from build123d import *

# Parameters (mm, degrees)
F0_W     = 80
F0_H     = 40
F1_DEPTH = 5
F2_W     = 80
F2_H     = 25
F2_R     = 3
F3_DEPTH = 5
F4_R     = 4.99999
F5_R     = 3
F6_DEPTH = 3


# Not quite as in the source:
# - a fillet or chamfer is up to 0.001 mm smaller than in the source, because OpenCascade refuses the exact size


with BuildPart() as f1:
    # F0 (on Top) → F1 (new body)
    with BuildSketch(Plane.XY):
        with Locations((-1.6386443377, -15.6908366084)):
            Rectangle(F0_W, F0_H)
    extrude(amount=-F1_DEPTH)

    # F2 (on face) → F3 (join)
    with BuildSketch(Plane.XZ.offset(35.6908366084)):
        with Locations((-1.6386443377, 12.5)):
            Rectangle(F2_W, F2_H)
        with Locations((-11.1386443377, 10)):
            Circle(F2_R, mode=Mode.SUBTRACT)
        with Locations((7.8613556623, 10)):
            Circle(F2_R, mode=Mode.SUBTRACT)
    extrude(amount=-F3_DEPTH)

    # F4 (radius 5 in the source; OpenCascade refuses exactly that, so slightly less here)
    f4_edges = [f1.edges().sort_by_distance(p)[0] for p in [
        (-41.638644, -33.190837, 25),
        (38.361356, -33.190837, 25),
        (-1.638644, 4.309163, 0),
    ]]
    fillet(f4_edges, radius=F4_R)

    # F5 (on face) → F6 (cut)
    with BuildSketch(Plane(origin=(0, -30.6908366084, 0), x_dir=(-1, 0, 0), z_dir=(0, 1, 0))):
        with BuildLine():
            ThreePointArc((-7.8613556623, 1.5), (-1.8509480223, 3.9895923599), (0.6386443377, 10))
            ThreePointArc((0.6386443377, 10), (-1.8509480223, 16.0104076401), (-7.8613556623, 18.5))
            ThreePointArc((-7.8613556623, 18.5), (-16.3613556623, 10), (-7.8613556623, 1.5))
        make_face()
        with Locations((-7.8613556623, 10)):
            Circle(F5_R, mode=Mode.SUBTRACT)
        with BuildLine():
            ThreePointArc((-7.8613556623, 18.5), (-1.8509480223, 16.0104076401), (0.6386443377, 10))
            ThreePointArc((0.6386443377, 10), (-1.8509480223, 3.9895923599), (-7.8613556623, 1.5))
            Line((-7.8613556623, 1.5), (11.1386443377, 1.5))
            ThreePointArc((11.1386443377, 1.5), (2.6386443377, 10), (11.1386443377, 18.5))
            Line((11.1386443377, 18.5), (-7.8613556623, 18.5))
        make_face()
        with BuildLine():
            ThreePointArc((19.6386443377, 10), (17.1490519777, 16.0104076401), (11.1386443377, 18.5))
            ThreePointArc((11.1386443377, 18.5), (2.6386443377, 10), (11.1386443377, 1.5))
            ThreePointArc((11.1386443377, 1.5), (17.1490519777, 3.9895923599), (19.6386443377, 10))
        make_face()
        with Locations((11.1386443377, 10)):
            Circle(F5_R, mode=Mode.SUBTRACT)
        with Locations((11.1386443377, 10)):
            Circle(F5_R)
        with Locations((-7.8613556623, 10)):
            Circle(F5_R)
    extrude(amount=-F6_DEPTH, mode=Mode.SUBTRACT)


solid = f1.part
Source: CAD feature listing. Evaluate the final solid. Frame: model axes, mm. A direction names the side the tool comes from. Round coordinates to 2 decimals unless told otherwise and drop trailing zeros. Loops run counter-clockwise (first coordinate to the right, second up) from the corner with the lowest first, then second, coordinate; pieces in that order, holes last.
Q1. Section A-A, the plane y = -32. Return loops of the section in (x, z).
Q2. First-contact query: P1, Ø24, axis at x = -11, y = -16.5, coming from the +Z side; P2, Ø5, axis at x = -2, z = 7.5, coming from the +Y side; P3, Ø4, axis at x = 8, z = 17, coming from the +Y side. Flat tips, straight axial feed; report the tip coordinate or a pass-through.
Q3. Mould query, pull axis Z, two halves, no side actions, for faces 4 (the face through (-2, -32, 18.5)), 5 (the face through (-1.08, 2.81, -1.43)), 6 (the face through (-41.639, -23, -1)). Classes: pulls with the +Z half, pulls with the -Z half, needs draft (parallel to the pull), parting line crosses it, or undercut.
Q4. Access query for faces 1 (the face through (-2, -15, 0)), 2 (the face through (-40.21, -33.16, 23.5)), 3 (the face through (-1, -33.691, 10)). Directions: +Z, -Z, +X, -X, +Y, -Y. A direction counts if a zero-diameter tool reaches every point of the face in a straight line with its end or side. Return the directions, or none.
Q5. Ray query, line 1 (Y direction, x = -24, z = 6.25); line 2 (Z direction, x = 12.5, y = -27.5); line 3 (Y direction, x = 5.5, z = 15.25). Return the intervals inside material, ascending.
Q6. Section D-D, the plane z = 14. Return loops of the section in (x, y).
Q7. Section C-C, the plane z = 9. Return loops of the section in (x, y), plus the area to 3 significant figures.
Solutions:
1. outline: (-41.64, -5) - (38.36, -5) - (38.36, 20) arc R5 ccw to (33.36, 25) - (-36.64, 25) arc R5 ccw to (-41.64, 20) - close; hole (-11.14, 1.5) - (7.86, 1.5) arc R8.5 ccw to (7.86, 18.5) - (-11.14, 18.5) arc R8.5 ccw to start
2. P1: stops at z = 0
2. P2: stops at y = -33.69
2. P3: stops at y = -30.69
3. face 4: undercut
3. face 5: pulls with the +Z half
3. face 6: needs draft
4. face 1: +Z, +X, -X, +Y
4. face 2: +Z, -X, +Y, -Y
4. face 3: +Y
5. line 1: y = -35.69 to -30.69
5. line 2: z = -5 to 0
5. line 3: y = -35.69 to -33.69
6. outline: (-41.64, -35.69) - (38.36, -35.69) - (38.36, -30.69) - (15.36, -30.69) - (15.36, -33.69) - (-18.64, -33.69) - (-18.64, -30.69) - (-41.64, -30.69) - close
7. outline: (-41.64, -35.69) - (-13.97, -35.69) - (-13.97, -33.69) - (-19.58, -33.69) - (-19.58, -30.69) - (-41.64, -30.69) - close; (-8.31, -35.69) - (5.03, -35.69) - (5.03, -33.69) - (-8.31, -33.69) - close; (10.69, -35.69) - (38.36, -35.69) - (38.36, -30.69) - (16.3, -30.69) - (16.3, -33.69) - (10.69, -33.69) - close
7. area: 270 mm2
